Geometry: final body of the model. Coordinates: model frame, mm. Give positions to 0.01 mm unless a question says otherwise; leave off trailing zeros. Write each loop counter-clockwise with the first axis right and the second up, starting at its lowest first coordinate (ties: lowest second). Pieces come first, ordered by that corner, then holes.
Q1. Cut plane A-A on z = 3.75. Return the cut outline in (x, y), plus the area to 3 significant figures.
Q2. Line query: L1, parallel to Y at x = 3, z = 3.5; L2, parallel to Y at x = 4.75, z = -8.75. Output: solid intervals per line, ascending.
Q3. Pin query (flat end, axial travel): pin 1 (0.5 mm diameter, centred on x = 5.5, z = -2.5, fed in from +Y); pin 2 (0.5 mm diameter, centred on x = 7.5, z = 0, fed in from +Y). Return the tip coordinate at first contact, or that it passes through.
```python
from build123d import *

# Parameters (mm, degrees)
EXTRUDE_1_DEPTH = 10


with BuildPart() as part:
    # 草图2 → 凸台-拉伸1 (new body)
    with BuildSketch(Plane(origin=(0, 0, 0), x_dir=(0, 0, -1), z_dir=(1, 0, 0))):
        Polygon((-10, 0), (10, 0), (10, 1.6), (9.6, 2), (9, 2), (8.6, 1.6), (8, 1.6), (7.6, 2), (7, 2), (6.6, 1.6), (6, 1.6), (5.6, 2), (5, 2), (4.6, 1.6), (4, 1.6), (3.6, 2), (3, 2), (2.6, 1.6), (2, 1.6), (1.6, 2), (1, 2), (0.6, 1.6), (0, 1.6), (-0.4, 2), (-1, 2), (-1.4, 1.6), (-2, 1.6), (-2.4, 2), (-3, 2), (-3.4, 1.6), (-4, 1.6), (-4.4, 2), (-5, 2), (-5.4, 1.6), (-6, 1.6), (-6.4, 2), (-7, 2), (-7.4, 1.6), (-8, 1.6), (-8.4, 2), (-9, 2), (-9.4, 1.6), (-10, 1.6), align=None)
    extrude(amount=EXTRUDE_1_DEPTH)


solid = part.part
```
Data:
1. outline: (0, 0) - (10, 0) - (10, 1.6) - (0, 1.6) - close
1. area: 16.0 mm2
2. L1: y = 0 to 1.6
2. L2: y = 0 to 1.75
3. pin 1: stops at y = 1.75
3. pin 2: stops at y = 1.85
